Design review of the part built by this model. Coordinates are the model's own, in mm. Give positions to 0.01 mm unless a question says otherwise; leave off trailing zeros. Loops run counter-clockwise (first coordinate to the right, second up) from the corner with the lowest first, then second, coordinate; pieces in that order, holes last. Notation, with made-up numbers: (18.25, -31) -> (39.25, -31) arc R27 cw to (39.25, 6) -> close; hole circle Ø8 at (-27.5, 37). An arc over 180 degrees is marked (long way). Use CSV: the item, a comma, the result in double quotes. Start each with the question number.
Item 1: We need section C-C (x = 329). State the section outline as (y, z) points.
Item 2: We need section A-A (z = 0). State the section outline as (x, y) points (3 decimals).
Item 3: Wall thickness on line 1 along X through (y, z) = (-25, 31); line 2 along X through (y, z) = (-4, 34.5); line 3 along Y through (x, z) = (378, 2): over which ranges is each line inside the solid? List them lowest first. Write a range as from..to.
Item 4: Clearance check with flat-ended pins moving along their axes: pin 1 (5 mm diameter, centred on x = 462.5, z = 9, fed in from +Y); pin 2 (3 mm diameter, centred on x = 532, y = 0, fed in from +Z); pin 3 (3 mm diameter, centred on x = 930.5, z = -6.5, fed in from -Y); pin 4 (5 mm diameter, centred on x = 535.5, z = -27, fed in from +Y). State where each tip first meets the part, or that it passes through.
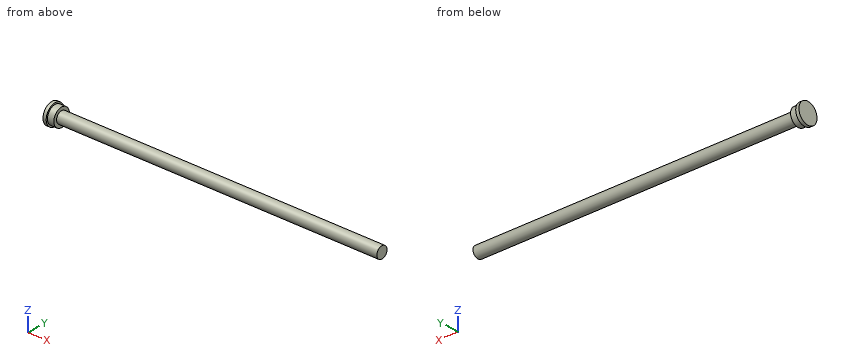
from build123d import *

# Parameters (mm, degrees)
SKETCH1_R           = 34.925
BOSS_EXTRUDE1_DEPTH = 25.4
SKETCH2_R           = 22.86
BOSS_EXTRUDE2_DEPTH = 1270
SKETCH3_R           = 40.64
BOSS_EXTRUDE3_DEPTH = 12.7


with BuildPart() as part:
    # Sketch1 → Boss-Extrude1 (new body)
    with BuildSketch(Plane(origin=(0, 0, 0), x_dir=(0, 0, -1), z_dir=(1, 0, 0))):
        Circle(SKETCH1_R)
    extrude(amount=BOSS_EXTRUDE1_DEPTH)

    # Sketch2 → Boss-Extrude2 (add)
    with BuildSketch(Plane(origin=(25.4, 0, 0), x_dir=(0, 0, -1), z_dir=(1, 0, 0))):
        Circle(SKETCH2_R)
    extrude(amount=BOSS_EXTRUDE2_DEPTH)

    # Sketch3 → Boss-Extrude3 (add)
    with BuildSketch(Plane.ZY):
        Circle(SKETCH3_R)
    extrude(amount=BOSS_EXTRUDE3_DEPTH)


solid = part.part
Results found:
1,outline,"circle Ø45.72 at (0, 0)"
2,outline,"(-12.7, -40.64) -> (0, -40.64) -> (0, -34.925) -> (25.4, -34.925) -> (25.4, -22.86) -> (1295.4, -22.86) -> (1295.4, 22.86) -> (25.4, 22.86) -> (25.4, 34.925) -> (0, 34.925) -> (0, 40.64) -> (-12.7, 40.64) -> close"
3,line 1,"-12.7..0"
3,line 2,"-12.7..25.4"
3,line 3,"-22.77..22.77"
4,pin 1,"y = 21.92"
4,pin 2,"z = 22.86"
4,pin 3,"y = -22.31"
4,pin 4,"through"
